Can you work these out from the model? Positions are in its coordinate system, mm. A direction names the side the tool comes from. Give positions to 0.01 mm unless a question says otherwise; leave off trailing zeros. Order: outer loops, then holes, each group sorted by start corner. A loop starts at its lowest first (then second) coordinate and runs counter-clockwise, first axis right, second up. Notation, with made-up numbers: (89.25, -12) - (109.25, -12) arc R17 cw to (109.25, 13) - close; hole circle Ø11 at (27.5, 12.5). An arc over 180 degrees is marked (long way). Return JSON: item names as keys, results as strings.
```python
from build123d import *

# Parameters (mm, degrees)
F0_W     = 623.337
F0_H     = 160
F1_DEPTH = 800
F2_T     = -19
F3_W     = 19
F3_H     = 25
F4_DEPTH = 800
F6_W     = 715.337
F6_H     = 211
F7_DEPTH = 19
F9_SIZE  = 8


with BuildPart() as f1:
    # F0 (on Front) → F1 (new body)
    with BuildSketch(Plane.XZ):
        with Locations((311.6685, 80)):
            Rectangle(F0_W, F0_H)
    extrude(amount=F1_DEPTH)

    # F2
    f2_openings = [f1.faces().sort_by_distance(p)[0] for p in [
        (311.6685, -400, 160),
    ]]
    offset(amount=F2_T, openings=f2_openings)


with BuildPart() as f4:
    # F3 (on face) → F4 (new body)
    with BuildSketch(Plane.XZ.offset(800)):
        with Locations((-9.5, 134.5)):
            Rectangle(F3_W, F3_H)
        with Locations((632.837, 134.5)):
            Rectangle(F3_W, F3_H)
    extrude(amount=-F4_DEPTH)


with BuildPart() as f1_1:
    add(f1.part)

    # F5: union F4
    add(f4.part)

    # F6 (on face) → F7 (join)
    with BuildSketch(Plane.XZ.offset(800)):
        with Locations((311.6685, 105.5)):
            Rectangle(F6_W, F6_H)
    extrude(amount=F7_DEPTH)

    # F9
    f9_edges = [f1_1.edges().sort_by_distance(p)[0] for p in [
        (311.6685, -800, 211),
    ]]
    chamfer(f9_edges, length=F9_SIZE)


solid = f1_1.part
```
1. Suppose I cut it at B-B (x = 475.5). List the corners of the cut face in (y, z) for me, plus the area to 3 significant figures.
Checks:
{"outline": "(-819, 0) - (0, 0) - (0, 160) - (-19, 160) - (-19, 19) - (-781, 19) - (-781, 160) - (-800, 160) - (-800, 203) - (-808, 211) - (-819, 211) - close", "area": "24,500 mm^2"}
2. Suppose I cut it at D-D (z = 69). List the corners of the cut face in (x, y) for me.
Checks:
{"outline": "(-46, -819) - (669.34, -819) - (669.34, -800) - (623.34, -800) - (623.34, 0) - (0, 0) - (0, -800) - (-46, -800) - close; hole (19, -781) - (604.34, -781) - (604.34, -19) - (19, -19) - close"}
3. Suppose I cut it at A-A (z = 131.5). List the corners of the cut face in (x, y) for me.
Checks:
{"outline": "(-46, -819) - (669.34, -819) - (669.34, -800) - (642.34, -800) - (642.34, 0) - (-19, 0) - (-19, -800) - (-46, -800) - close; hole (19, -781) - (604.34, -781) - (604.34, -19) - (19, -19) - close"}
4. On a 3-axis mill with a long thin cutter (end or side, diameter ignored), from which of +Z, -Z, +X, -X, +Y, -Y can I reach the whole of each face in a straight line? I mean faces 1 (the face through (-10, -406, 147)), 2 (the face through (0, -394, 60)), 3 (the face through (19, -395, 89)), 4 (the face through (633, -406, 147)). Say none if no direction works.
Checks:
{"face 1": "+Z, -X, +Y", "face 2": "-Z, -X, +Y", "face 3": "+Z", "face 4": "+Z, +X, +Y"}
5. Suppose I cut it at C-C (y = -501). List the corners of the cut face in (x, z) for me, plus the area to 3 significant figures.
Checks:
{"outline": "(-19, 122) - (0, 122) - (0, 0) - (623.34, 0) - (623.34, 122) - (642.34, 122) - (642.34, 147) - (623.34, 147) - (623.34, 160) - (604.34, 160) - (604.34, 19) - (19, 19) - (19, 160) - (0, 160) - (0, 147) - (-19, 147) - close", "area": "18,200 mm^2"}
6. Thinking about a two-plate mould opening in Y: for faces 5 (the face through (308, -19, 90)), 6 (the face through (308, -781, 90)), 7 (the face through (307, -819, 107)), 8 (the face through (-19, -406, 134)), which applies, +Y half, -Y half, draft (parallel to the pull), parting line (faces both ways), or undercut?
Checks:
{"face 5": "undercut", "face 6": "undercut", "face 7": "-Y half", "face 8": "draft"}
7. If I drill on L1, parallel to Y at x = 273.5, z = 82.5; L2, parallel to X at y = -286, z = 58; L3, parallel to Z at x = 277, y = -627, over which ranges is the centre line in solid material (lowest first)? Write a range as [from, to].
Checks:
{"L1": "[-819, -781], [-19, 0]", "L2": "[0, 19], [604.34, 623.34]", "L3": "[0, 19]"}
8. For pin 1 Ø7.5 at (y, z) = (-410, 136.5) entering from +X; pin 2 Ø21 at (x, y) = (637, -275.5) entering from +Z; pin 3 Ø12.5 at (y, z) = (-271.5, 137.5) entering from -X, each with a flat end and sliding along its axis, tell me the tip position at first contact or that it passes through.
Checks:
{"pin 1": "x = 642.34", "pin 2": "z = 147", "pin 3": "x = -19"}
